Here's the drawing with two shaded views (mm, measured from the low corner). I have some questions. Coordinates: 2 decimals unless noted, no trailing zeros. Write each loop counter-clockwise with the first axis right and the second up, starting at its lowest first coordinate (ties: lowest second). Pieces come first, ordered by that corner, then holes.
Item 1: I'm going to push flat-ended pins straight in: pin 1 Ø4 at (y, z) = (5, 11) entering from -X; pin 2 Ø3 at (y, z) = (1.5, 3.5) entering from +X; pin 3 Ø6 at (y, z) = (5.5, 2.5) entering from +X. Where does each tip first touch, or does it pass through?
Item 2: If we section it at B-B (x = 8): Please give me the cut outline in (y, z), then the cut area to 3 significant figures.
Item 3: If we section it at D-D (z = 7.75): Please give me the cut outline in (x, y).
Item 4: If we section it at C-C (z = 4.75): Please give me the cut outline in (x, y), then the cut area to 3 significant figures.
Item 5: If we section it at A-A (y = 3.5): Count the separate pieces of the cut face and the enclosed holes in it, then the cut area to 3 significant figures.
Item 6: If I drill on line 1 (X direction, y = 7.5, z = 6); line 2 (X direction, y = 8.5, z = 3.5) (1 decimal); line 3 (Z direction, x = 46, y = 2), over which ranges is the centre line in solid material (lowest first)?
Item 7: We'd pull the mould along Z, two halves only. Please class the marked faces 1, 2 and 3: +Z half, -Z half, draft (parallel to the pull), parting line (faces both ways), or undercut.
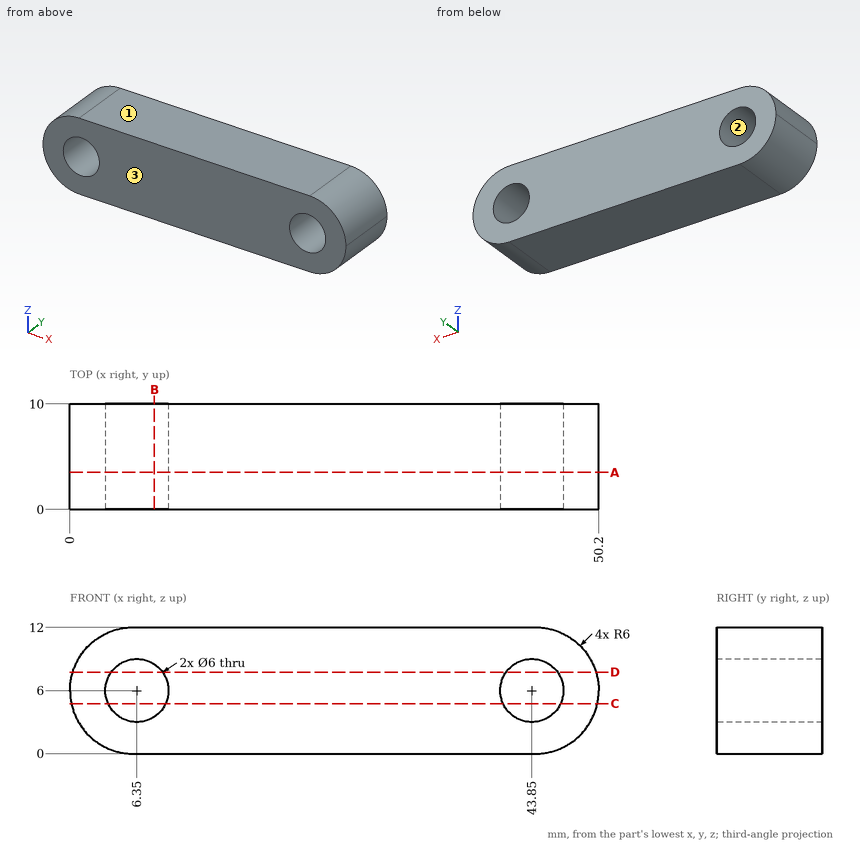
Answer list:
1. pin 1: stops at x = 0.8
1. pin 2: stops at x = 50.12
1. pin 3: stops at x = 50.18
2. outline: (0, 0) - (10, 0) - (10, 3.49) - (0, 3.49) - close; (0, 8.51) - (10, 8.51) - (10, 12) - (0, 12) - close
2. area: 69.9 mm2
3. outline: (0.26, 0) - (3.91, 0) - (3.91, 10) - (0.26, 10) - close; (8.79, 0) - (41.41, 0) - (41.41, 10) - (8.79, 10) - close; (46.29, 0) - (49.94, 0) - (49.94, 10) - (46.29, 10) - close
4. outline: (0.13, 0) - (3.62, 0) - (3.62, 10) - (0.13, 10) - close; (9.08, 0) - (41.12, 0) - (41.12, 10) - (9.08, 10) - close; (46.58, 0) - (50.07, 0) - (50.07, 10) - (46.58, 10) - close
4. area: 390 mm2
5. separate pieces: 1
5. enclosed holes: 2
5. area: 515 mm2
6. line 1: x = 0 to 3.35, 9.35 to 40.85, 46.85 to 50.2
6. line 2: x = 0.5 to 4.7, 8 to 42.2, 45.5 to 49.7
6. line 3: z = 0.28 to 3.91, 8.09 to 11.72
7. face 1: +Z half
7. face 2: undercut
7. face 3: draft
